Could you check a few things on this drawing? It's one solid part, dimensions in mm from its lowest x, y, z. A direction names the side the tool comes from. Give positions to 0.01 mm unless a question says otherwise; leave off trailing zeros. Order: outer loops, then holes, each group sorted by start corner. A loop starts at its lowest first (then second) coordinate and runs counter-clockwise, first axis right, second up. Notation, with made-up numbers: (-25, 46.25) - (-21, 46.25) arc R9 cw to (-21, 52.25) - close; hole circle Ø9 at (75.5, 14.25). An arc over 180 degrees is marked (long way). Put each result on its own line as item: value.
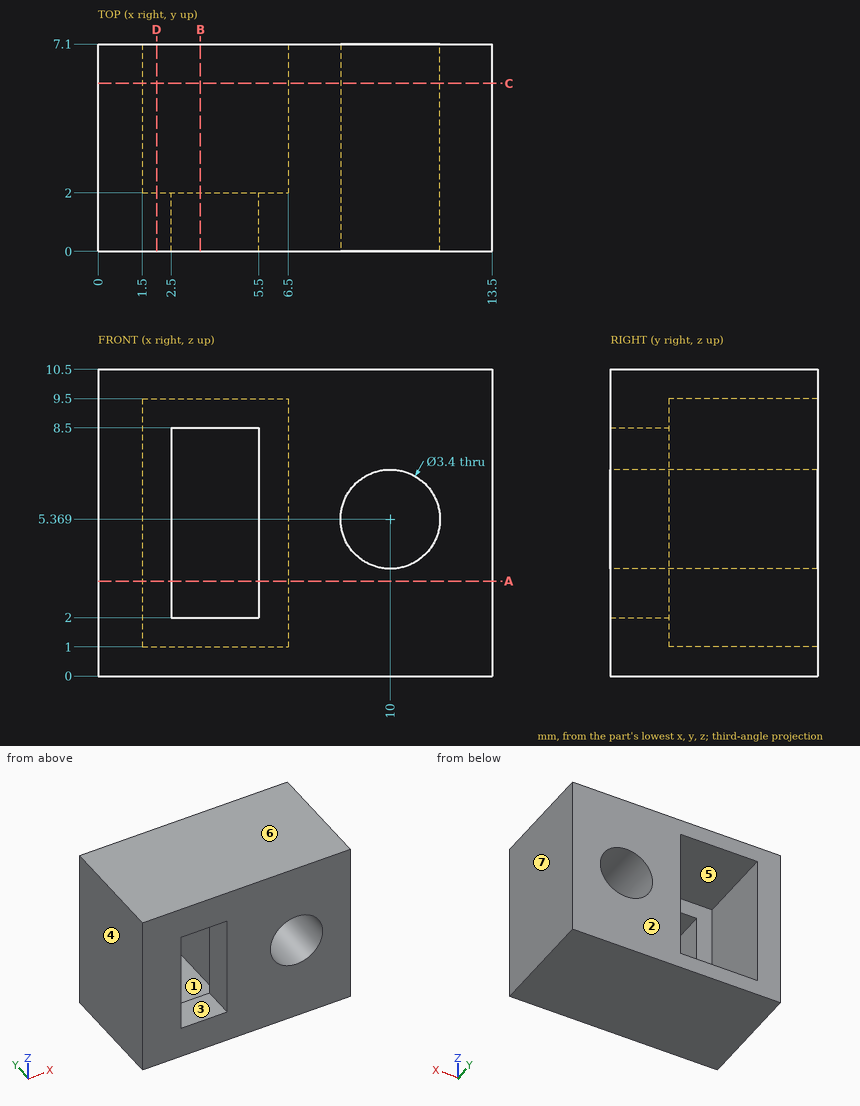
1) If I drill on line 1 (Z direction, x = 5, y = 5.5); line 2 (Z direction, x = 10, y = 4.5); line 3 (X direction, y = 6.75, z = 9.25), over which ranges is the centre line in solid material (lowest first)? Write a range as [from, to].
Filled in:
line 1: z = [0, 1], [9.5, 10.5]
line 2: z = [0, 3.67], [7.07, 10.5]
line 3: x = [0, 1.5], [6.5, 13.5]
2) Suppose I cut it at A-A, the plane z = 3.25. List the corners of the cut face in (x, y) for me.
Filled in:
outline: (0, 0) - (2.5, 0) - (2.5, 2) - (1.5, 2) - (1.5, 7.1) - (0, 7.1) - close; (5.5, 0) - (13.5, 0) - (13.5, 7.1) - (6.5, 7.1) - (6.5, 2) - (5.5, 2) - close
3) We'd pull the mould along X, two halves only. Please class the marked faces 4, 5, 6 and 7: pulls with the +X half, pulls with the -X half, needs draft (parallel to the pull), parting line crosses it, or undercut.
Filled in:
face 4: pulls with the -X half
face 5: undercut
face 6: needs draft
face 7: pulls with the +X half
4) Suppose I cut it at D-D, the plane x = 2. List the corners of the cut face in (y, z) for me, and give its area (3 significant figures).
Filled in:
outline: (0, 0) - (7.1, 0) - (7.1, 1) - (2, 1) - (2, 9.5) - (7.1, 9.5) - (7.1, 10.5) - (0, 10.5) - close
area: 31.2 mm^2
5) Suppose I cut it at B-B, the plane x = 3.5. List the corners of the cut face in (y, z) for me, and give its area (3 significant figures).
Filled in:
outline: (0, 0) - (7.1, 0) - (7.1, 1) - (2, 1) - (2, 2) - (0, 2) - close; (0, 8.5) - (2, 8.5) - (2, 9.5) - (7.1, 9.5) - (7.1, 10.5) - (0, 10.5) - close
area: 18.2 mm^2
6) Which directions (+Z, -Z, +X, -X, +Y, -Y) give clear straight access to the entire face, cutting with the end or side of a thin tool? Please do the marked faces 1, 2 and 3.
Filled in:
face 1: +Y
face 2: +Z, -Z, +X, -X, +Y
face 3: +Y, -Y
7) Suppose I cut it at C-C, the plane y = 5.75. List the corners of the cut face in (x, z) for me.
Filled in:
outline: (0, 0) - (13.5, 0) - (13.5, 10.5) - (0, 10.5) - close; hole (1.5, 1) - (6.5, 1) - (6.5, 9.5) - (1.5, 9.5) - close; hole circle Ø3.4 at (10, 5.37)
